Geometry: final body of the model. Coordinates: model frame, mm. Face numbers are marked on the shaded views. A direction names the side the tool comes from. Coordinates: 2 decimals unless noted, no trailing zeros. Loops run counter-clockwise (first coordinate to the right, second up) from the corner with the lowest first, then second, coordinate; pieces in that order, holes last. Notation, with made-up numbers: (-23, -32) - (20, -32) arc R21 ccw to (20, 1) - close; hole circle Ø7 at (19, 22). An arc over 180 degrees is marked (long way). Put each result on its own line as item: value. Start each with the question number.
1) Section B-B on z = -43. Output: boundary loops of the cut face in (x, y).
2) Contact query for flat-ended pins moving along their axis: pin 1 Ø1.5 at (x, z) = (-3.5, -13.5) entering from +Y; pin 2 Ø6 at (y, z) = (2.5, -7) entering from -X; pin 3 Ø4 at (x, z) = (-2, -25.5) entering from +Y. Output: stop coordinate, or through.
3) Material intervals for line 1 along Z through (x, y) = (1.25, -4); line 2 along Y through (x, z) = (0.25, -16); line 3 along Z through (x, y) = (-1.75, -2.25), sorted ascending. Write a range as from..to.
4) Reachability of the marked faces 1 and 2 from +Z, -Z, +X, -X, +Y, -Y: full face, straight path, thin tool, end or side. Return the list, or none.
5) Section A-A on y = 0. Output: boundary loops of the cut face in (x, z).
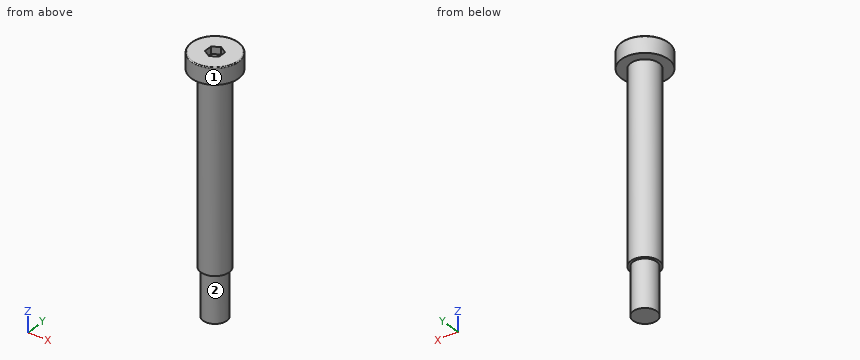
```python
from build123d import *

# Parameters (mm, degrees)
CUT_EXTRUDE_1_DEPTH = 1.5
FILLET_1_R          = 0.2


with BuildPart() as part:
    # 草图1 → 旋转1 (revolve)
    with BuildSketch(Plane(origin=(0, 0, 0), x_dir=(0, 0, -1), z_dir=(1, 0, 0))):
        Polygon((0, 0), (0, 5), (3.5, 5), (3.5, 3), (43.5, 3), (43.5, 2.5), (53.5, 2.5), (53.5, 0), align=None)
    revolve(axis=Axis((0, 0, -53.5), (0, 0, 1)))

    # 草图2 → 切除-拉伸1 (cut)
    with BuildSketch(Plane.XY):
        Polygon((1.5, 0.866025404), (0, 1.732050808), (-1.5, 0.866025404), (-1.5, -0.866025404), (0, -1.732050808), (1.5, -0.866025404), align=None)
    extrude(amount=-CUT_EXTRUDE_1_DEPTH, mode=Mode.SUBTRACT)

    # 圆角1
    fillet_1_edges = [part.edges().sort_by_distance(p)[0] for p in [
        (0, -5, 0),
    ]]
    fillet(fillet_1_edges, radius=FILLET_1_R)


solid = part.part
```
Answer block:
1. outline: circle Ø6 at (0, 0)
2. pin 1: stops at y = 1.2
2. pin 2: stops at x = -3
2. pin 3: stops at y = 3
3. line 1: z = -3.5..0
3. line 2: y = -2.99..2.99
3. line 3: z = -43.5..0
4. face 1: +Z, -Z
4. face 2: -Z
5. outline: (-5, -3.5) - (-3, -3.5) - (-3, -43.5) - (-2.5, -43.5) - (-2.5, -53.5) - (2.5, -53.5) - (2.5, -43.5) - (3, -43.5) - (3, -3.5) - (5, -3.5) - (5, -0.2) arc R0.2 ccw to (4.8, 0) - (1.5, 0) - (1.5, -1.5) - (-1.5, -1.5) - (-1.5, 0) - (-4.8, 0) arc R0.2 ccw to (-5, -0.2) - close
